Read the model definition and answer for the solid it produces. Units are mm, in the model's axes. Face numbers are marked on the shaded views. A direction names the side the tool comes from. Coordinates: 2 decimals unless noted, no trailing zeros. Write each loop counter-clockwise with the first axis right and the second up, starting at its lowest first coordinate (ties: lowest second). Pieces come first, ordered by that corner, then holes.
from build123d import *

# Parameters (mm, degrees)
BOSS_EXTRUDE1_DEPTH        = 66
CUT_EXTRUDE1_DEPTH         = 67.0000001
M3_5_CLEARANCE_HOLE1_D     = 4.199808185
M3_5_CLEARANCE_HOLE1_DEPTH = 66.000055
M3_5_CLEARANCE_HOLE2_D     = 3.949622561
M3_5_CLEARANCE_HOLE2_DEPTH = 66.000055
FILLET1_R                  = 5.024738629
FILLET2_R                  = 19.924521471
FILLET3_R                  = 74.958538247
BOSS_EXTRUDE2_DEPTH        = 45


with BuildPart() as part:
    # Sketch1 → Boss-Extrude1 (new body)
    with BuildSketch(Plane(origin=(0, 6, 0), x_dir=(1, 0, 0), z_dir=(0, 1, 0))):
        with BuildLine():
            Line((118.094019457, 109.999994984), (-118.094002078, 109.999994984))
            Line((-118.094002078, 109.999994984), (-159.951896595, 37.499994984))
            add(Edge.make_bspline(
                [(-159.951896595, 37.499994984), (-162.089834317, 33.796773054), (-165.842582605, 25.786056062), (-169.244504237, 13.08991169), (-169.999887381, 4.276053128), (-169.999989967, 0)],
                knots=[5.759586536, 5.759586536, 5.759586536, 5.759586536, 5.930628798, 6.11214304, 6.283185303, 6.283185303, 6.283185303, 6.283185303], degree=3))
            add(Edge.make_bspline(
                [(-169.999989967, 0), (-169.999887381, -4.276053128), (-169.244504237, -13.089911689), (-165.842582605, -25.786056062), (-162.089834317, -33.796773054), (-159.951896595, -37.499994984)],
                knots=[4e-09, 4e-09, 4e-09, 4e-09, 0.171042267, 0.352556509, 0.523598771, 0.523598771, 0.523598771, 0.523598771], degree=3))
            Line((-159.951896595, -37.499994984), (-90.801270189, -157.27241336))
            Line((-90.801270189, -157.27241336), (90.801270189, -157.27241336))
            Line((90.801270189, -157.27241336), (159.951905284, -37.5))
            add(Edge.make_bspline(
                [(159.951905284, -37.5), (162.089843006, -33.79677807), (165.842591294, -25.786061079), (169.244512926, -13.089916706), (169.99989607, -4.276058145), (169.999998656, -5.016e-06)],
                knots=[2.617993882, 2.617993882, 2.617993882, 2.617993882, 2.789036145, 2.970550387, 3.141592649, 3.141592649, 3.141592649, 3.141592649], degree=3))
            add(Edge.make_bspline(
                [(169.999998656, -5.016e-06), (169.99989607, 4.276048112), (169.244512926, 13.089906673), (165.842591294, 25.786051046), (162.089843006, 33.796768038), (159.951905284, 37.499989968)],
                knots=[3.141592658, 3.141592658, 3.141592658, 3.141592658, 3.31263492, 3.494149162, 3.665191425, 3.665191425, 3.665191425, 3.665191425], degree=3))
            Line((159.951905284, 37.499989968), (118.094019457, 109.999994984))
        make_face()
    extrude(amount=-BOSS_EXTRUDE1_DEPTH)

    # Sketch2 → Cut-Extrude1 (cut, through all)
    with BuildSketch(Plane.XZ.offset(60)):
        Polygon((3.5, -110), (3.5, -93), (30, -93), (30, -79), (-30, -79), (-30, -93), (-3.5, -93), (-3.5, -110), align=None)
    extrude(amount=-CUT_EXTRUDE1_DEPTH, mode=Mode.SUBTRACT)

    # M3.5 Clearance Hole1
    with Locations(Plane(origin=(0, -60, 0), x_dir=(-1, 0, 0), z_dir=(0, -1, 0))):
        with Locations((0, -0.001547229), (-97.9932, 0.001547229), (97.9932, 0.001547229), (120, 55.001547229), (-120, 55.001547229)):
            Hole(M3_5_CLEARANCE_HOLE1_D / 2, depth=M3_5_CLEARANCE_HOLE1_DEPTH)

    # M3.5 Clearance Hole2
    with Locations(Plane(origin=(0, -60, 0), x_dir=(-1, 0, 0), z_dir=(0, -1, 0))):
        with Locations((98, 102.43824134), (0, -109.21995866), (98, -109.21995866), (-98, -109.21995866), (111.4552, 69.84995866), (111.4552, -4.134e-05), (-111.4552, 69.84995866), (-111.4552, -4.134e-05), (-120, -55.00004134), (120, -55.00004134), (131.4, 50.30004134), (-131.4, 50.30004134), (131.4, -70.19995866), (-131.4, -70.19995866), (131.4, 63.00004134), (-131.4, 63.00004134), (131.4, -57.49995866), (-131.4, -57.49995866), (15, 101.50004134), (-98, 102.43824134), (-15, 101.50004134), (150.47, 38.10004134), (150.47, -38.09995866), (-150.47, 38.10004134), (-150.47, -38.09995866), (-82, -119.99995866), (82, -119.99995866)):
            Hole(M3_5_CLEARANCE_HOLE2_D / 2, depth=M3_5_CLEARANCE_HOLE2_DEPTH)

    # Fillet1
    fillet1_edges = [part.edges().sort_by_distance(p)[0] for p in [
        (-3.5, -27, -109.999994984),
        (-30, -27, -79),
        (30, -27, -79),
        (3.5, -27, -109.999994984),
        (-30, -27, -93),
        (-3.5, -27, -93),
        (30, -27, -93),
        (3.5, -27, -93),
    ]]
    fillet(fillet1_edges, radius=FILLET1_R)

    # Fillet2
    fillet2_edges = [part.edges().sort_by_distance(p)[0] for p in [
        (118.094019457, -27, -109.999994984),
        (-118.094002078, -27, -109.999994984),
    ]]
    fillet(fillet2_edges, radius=FILLET2_R)

    # Fillet3
    fillet3_edges = [part.edges().sort_by_distance(p)[0] for p in [
        (-90.801270189, -27, 157.27241336),
        (90.801270189, -27, 157.27241336),
    ]]
    fillet(fillet3_edges, radius=FILLET3_R)

    # Sketch7 → Boss-Extrude2 (add)
    with BuildSketch(Plane(origin=(0, 6, 0), x_dir=(1, 0, 0), z_dir=(0, 1, 0))):
        with BuildLine():
            Line((-16.390788815, -41.267338357), (-16.410904507, -52.265499005))
            ThreePointArc((-16.410904507, -52.265499005), (-15.908890548, -53.485611522), (-14.690365147, -53.991465667))
            Line((-14.690365147, -53.991465667), (11.309634853, -53.991465667))
            ThreePointArc((11.309634853, -53.991465667), (12.528160254, -53.485611522), (13.030174213, -52.265499005))
            Line((13.030174213, -52.265499005), (13.010058521, -41.267338357))
            ThreePointArc((13.010058521, -41.267338357), (12.514864968, -40.042764602), (11.309634853, -39.50219277))
            Line((11.309634853, -39.50219277), (-14.690365147, -39.50219277))
            ThreePointArc((-14.690365147, -39.50219277), (-15.915842564, -40.023259701), (-16.390788815, -41.267338357))
        make_face()
    extrude(amount=BOSS_EXTRUDE2_DEPTH)


solid = part.part
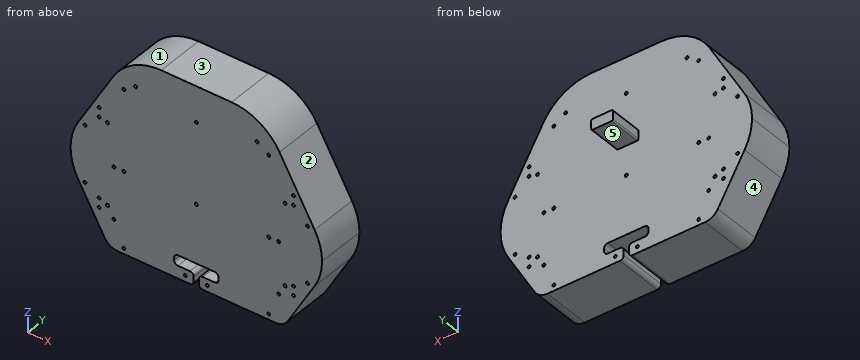
Item 1: Determine the mould class of the marked faces 1, 2 and 3 for opening direction X: +X half, -X half, draft (parallel to the pull), parting line (faces both ways), or undercut.
Item 2: The part is cut by section A-A (y = 25.5). Give the vertices of the cut face in (x, z).
Item 3: Find the intervals of material crossed by probe 1 along Z at (x, y) = (-98, -29.5); probe 2 along Z at (x, y) = (130.5, -37); probe 3 along Z at (x, y) = (-150.47, -20), in increasing order.
Item 4: For the marked faces 4 and 5, determine the directions among +Z, -Z, +X, -X, +Y, -Y from which every point of the face is accessible in a straight line to the end or side of a thin tool.
Item 5: The part is cut by section D-D (y = -12). State how many separate pieces and enclosed holes the cut face has, and give its area (3 significant figures).
Item 6: The part is cut by section C-C (z = 131.5). Give the vertices of the cut face in (x, y).
Item 7: Given pin 1 (6.5 mm diameter, centred on x = 98, z = -102.44, fed in from +Y); pin 2 (3 mm diameter, centred on y = -11, z = -85, fed in from -X); pin 3 (10 mm diameter, centred on x = -134, z = 96, fed in from +Y); pin 4 (6.5 mm diameter, centred on x = 0, z = 0, fed in from -Y), each flat-ended and moving along its own axis, determine where each tip first touches the part or whether it passes through.
Item 8: The part is cut by section B-B (x = 38.5). Give the vertices of the cut face in (y, z).
Answer:
1. face 1: -X half
1. face 2: +X half
1. face 3: draft
2. outline: (-16.41, 52.27) - (-16.39, 41.27) arc R1.7 ccw to (-14.69, 39.5) - (11.31, 39.5) arc R1.77 ccw to (13.01, 41.27) - (13.03, 52.27) arc R1.72 ccw to (11.31, 53.99) - (-14.69, 53.99) arc R1.72 ccw to start
3. probe 1: z = -110 to -104.41, -100.46 to -2.1, 2.1 to 107.25, 111.19 to 137.73
3. probe 2: z = -88.51 to -64.76, -61.24 to -52.06, -48.54 to 55.74, 59.26 to 68.44, 71.96 to 88.51
3. probe 3: z = -53.92 to -40.07, -36.13 to 36.13, 40.07 to 53.92
4. face 4: -Z, -X, +Y, -Y
4. face 5: -Z, +X, -X, +Y
5. separate pieces: 1
5. enclosed holes: 32
5. area: 73,200 mm2
6. outline: (-104.09, -60) - (104.09, -60) - (104.09, 6) - (-104.09, 6) - close
7. pin 1: stops at y = 6
7. pin 2: stops at x = -133.39
7. pin 3: passes through
7. pin 4: stops at y = -60
8. outline: (-60, -110) - (6, -110) - (6, 157.27) - (-60, 157.27) - close
